Could you check a few things on this model? Use its own coordinates, in mm. Give positions to 0.01 mm unless a question says otherwise; leave off trailing zeros. Loops run counter-clockwise (first coordinate to the right, second up) from the corner with the lowest first, then second, coordinate; pieces in that order, holes last. Notation, with made-up numbers: M -21.75,-26.75 L 34.25,-26.75 A14 ccw 34.25,-12.75 Z; hole C -33.5,-4 d1. An arc over 180 degrees is marked long. Write each question's results on one line, items separated by ' | '. Start each with the question number.
from build123d import *

# Parameters (mm, degrees)
SKETCH1_R           = 2.55
BOSS_EXTRUDE1_DEPTH = 12.7


with BuildPart() as part:
    # Sketch1 → Boss-Extrude1 (new body)
    with BuildSketch(Plane.XY):
        with BuildLine():
            Line((59.789213932, 216.60923387), (59.789213932, 206.609233872))
            Line((59.789213932, 206.609233872), (72.963032743, 206.609233872))
            ThreePointArc((72.963032743, 206.609233872), (73.789213933, 206.834833872), (74.615395122, 206.609233872))
            Line((74.615395122, 206.609233872), (93.963032742, 206.609233872))
            ThreePointArc((93.963032742, 206.609233872), (94.789213933, 206.834833872), (95.615395124, 206.609233871))
            Line((95.615395124, 206.609233871), (145.789213933, 206.609233871))
            ThreePointArc((145.789213933, 206.609233871), (155.789213933, 216.609233871), (145.789213933, 226.609233871))
            Line((145.789213933, 226.609233871), (95.615395124, 226.609233871))
            ThreePointArc((95.615395124, 226.609233871), (94.789213933, 226.38363387), (93.963032742, 226.60923387))
            Line((93.963032742, 226.60923387), (74.615395122, 226.60923387))
            ThreePointArc((74.615395122, 226.60923387), (73.789213933, 226.38363387), (72.963032743, 226.60923387))
            Line((72.963032743, 226.60923387), (69.789213932, 226.60923387))
            ThreePointArc((69.789213932, 226.60923387), (62.71814612, 223.680301682), (59.789213932, 216.60923387))
        make_face()
        with Locations((144.789213934, 216.609233872)):
            Circle(SKETCH1_R, mode=Mode.SUBTRACT)
    extrude(amount=BOSS_EXTRUDE1_DEPTH)


solid = part.part
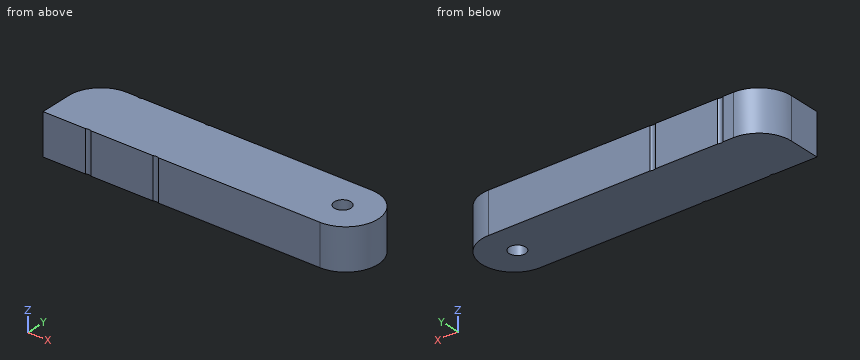
1) Please list where these lines run through material, in increasing order: line 1 (X direction, y = 218.5, z = 10); line 2 (Y direction, x = 95, z = 2); line 3 (X direction, y = 212, z = 1.5). Write a range as from..to.
2) If we section it at A-A on z = 10: Write out the boundary of the cut face in (x, y), plus the area to 3 significant figures.
3) If we section it at B-B on y = 215.25: Write out the boundary of the cut face in (x, z).
4) If we section it at D-D on y = 209.5: Write out the boundary of the cut face in (x, z), plus the area to 3 significant figures.
5) If we section it at C-C on y = 224: Write out the boundary of the cut face in (x, z), plus the area to 3 significant figures.
6) I'm going to push a flat-ended pin straight in: P1, Ø1.5, axis at x = 88, y = 209, coming from the -Z side. Where does the tip first touch, or does it pass through?
Calculated:
1) line 1: x = 59.97..143.08, 146.5..155.61 | line 2: y = 206.82..226.4 | line 3: x = 59.79..154.66
2) outline: M 59.79,206.61 L 72.96,206.61 A1.63 cw 74.62,206.61 L 93.96,206.61 A1.63 cw 95.62,206.61 L 145.79,206.61 A10 ccw 145.79,226.61 L 95.62,226.61 A1.63 cw 93.96,226.61 L 74.62,226.61 A1.63 cw 72.96,226.61 L 69.79,226.61 A10 ccw 59.79,216.61 Z; hole C 144.79,216.61 d5.1 | area: 1,830 mm2
3) outline: M 59.79,0 L 142.63,0 L 142.63,12.7 L 59.79,12.7 Z; M 146.95,0 L 155.7,0 L 155.7,12.7 L 146.95,12.7 Z
4) outline: M 59.79,0 L 152.82,0 L 152.82,12.7 L 59.79,12.7 Z | area: 1,180 mm2
5) outline: M 63.05,0 L 152.53,0 L 152.53,12.7 L 63.05,12.7 Z | area: 1,140 mm2
6) P1: stops at z = 0
